```python
from build123d import *

# Parameters (mm, degrees)
SKETCH2_R           = 3.4
BOSS_EXTRUDE1_DEPTH = 8
SKETCH3_R           = 3.4
BOSS_EXTRUDE2_DEPTH = 2
BOSS_EXTRUDE3_DEPTH = 14


with BuildPart() as part:
    # Sketch2 → Boss-Extrude1 (new body)
    with BuildSketch(Plane.XY):
        Circle(SKETCH2_R)
        with BuildLine():
            Line((-1.7, -1.316244658), (-1.7, 1.316244658))
            ThreePointArc((-1.7, 1.316244658), (2.15, 0), (-1.7, -1.316244658))
        make_face(mode=Mode.SUBTRACT)
    extrude(amount=BOSS_EXTRUDE1_DEPTH)

    # Sketch3 → Boss-Extrude2 (add)
    with BuildSketch(Plane.XY.offset(8)):
        Circle(SKETCH3_R)
    extrude(amount=BOSS_EXTRUDE2_DEPTH)

    # Sketch4 → Boss-Extrude3 (add)
    with BuildSketch(Plane.XY.offset(10)):
        with BuildLine():
            Line((-2.8, -1.7), (-2.8, 1.7))
            ThreePointArc((-2.8, 1.7), (0, 3.275667871), (2.8, 1.7))
            Line((2.8, 1.7), (2.8, -1.7))
            ThreePointArc((2.8, -1.7), (0, -3.275667871), (-2.8, -1.7))
        make_face()
    extrude(amount=BOSS_EXTRUDE3_DEPTH)


solid = part.part
```
For this review, take the finished solid that the model builds, in its own axes (mm). A direction names the side the tool comes from. Coordinates: 2 decimals unless noted, no trailing zeros. Loops run counter-clockwise (first coordinate to the right, second up) from the corner with the lowest first, then second, coordinate; pieces in that order, holes last. Notation, with made-up numbers: (15.5, 3.5) -> (20.5, 3.5) arc R30 cw to (20.5, 42.5) -> close; hole circle Ø11 at (68, 28.25). An arc over 180 degrees is marked (long way). Return JSON: item names as keys, results as strings. Group by question number.
(1) For pin 1 Ø1.7 at (y, z) = (0, 15.5) entering from -X; pin 2 Ø1 at (y, z) = (-0.5, 15.5) entering from +X; pin 3 Ø3 at (x, z) = (-2.5, 20.5) entering from -Y, all flat-tipped, find the tip position at first contact; note any pin that passes through.
(2) Consider section A-A, the plane z = 4.5. Give the boundary of the cut face in (x, y).
(3) Consider section D-D, the plane z = 21.25. Give the boundary of the cut face in (x, y).
(4) Mouldability with a two-part tool opening along Y and no side actions: class faces 4 (the flat face through (3, 0, 10)), 5 (the cylindrical face through (-0.74, -3.32, 4.93)), 6 (the flat face through (-1.7, 0, 4)) as pulls with the +Y half, pulls with the -Y half, needs draft (parallel to the pull), parting line crosses it, or undercut.
(5) Consider section C-C, the plane y = 0. Give the boundary of the cut face in (x, z), plus the area to 3 significant figures.
(6) Consider section B-B, the plane x = 0. Give the boundary of the cut face in (y, z).
(7) Tool access review of faces 1 (the cylindrical face through (-0.047, 3.275, 16.902)), 2 (the flat face through (2.8, 0, 17)), 3 (the flat face through (0, 0, 8)): name each direction out of +Z, -Z, +X, -X, +Y, -Y from which nothing blocks a thin tool from reaching the whole face with its end or side.
(8) To check wall thickness, follow L1, parallel to Y at x = 0, z = 4.5; L2, parallel to Z at x = 0.25, y = -0.25; L3, parallel to X at y = -0.75, z = 14.5. State the ranges of each line that lie inside material, in increasing order.
Results below:
{
 "1": {"pin 1": "stops at x = -2.8", "pin 2": "stops at x = 2.8", "pin 3": "stops at y = -3.12"},
 "2": {"outline": "circle Ø6.8 at (0, 0); hole (-1.7, -1.32) arc R2.15 ccw (long way) to (-1.7, 1.32) -> close"},
 "3": {"outline": "(-2.8, -1.7) arc R3.28 ccw to (2.8, -1.7) -> (2.8, 1.7) arc R3.28 ccw to (-2.8, 1.7) -> close"},
 "4": {"face 4": "needs draft", "face 5": "parting line crosses it", "face 6": "undercut"},
 "5": {"outline": "(-3.4, 0) -> (-1.7, 0) -> (-1.7, 8) -> (2.15, 8) -> (2.15, 0) -> (3.4, 0) -> (3.4, 10) -> (2.8, 10) -> (2.8, 24) -> (-2.8, 24) -> (-2.8, 10) -> (-3.4, 10) -> close", "area": "116 mm2"},
 "6": {"outline": "(-3.4, 0) -> (-2.15, 0) -> (-2.15, 8) -> (2.15, 8) -> (2.15, 0) -> (3.4, 0) -> (3.4, 10) -> (3.28, 10) -> (3.28, 24) -> (-3.28, 24) -> (-3.28, 10) -> (-3.4, 10) -> close"},
 "7": {"face 1": "+Z, +Y", "face 2": "+Z, +X, +Y, -Y", "face 3": "-Z"},
 "8": {"L1": "y = -3.4 to -2.15, 2.15 to 3.4", "L2": "z = 8 to 24", "L3": "x = -2.8 to 2.8"}
}
